from build123d import *

# Parameters (mm, degrees)
F1_DEPTH = 3.81
F3_DEPTH = 2.54
F5_DEPTH = 1.905


with BuildPart() as f1:
    # F0 (on Front) → F1 (new body)
    with BuildSketch(Plane.XZ):
        Polygon((-217.349024, 262.862362), (-255.449024, 262.862362), (-267.222571, 299.097615), (-278.996119, 262.862362), (-317.096119, 262.862362), (-286.272571, 240.467744), (-298.046119, 204.23249), (-267.222571, 226.627108), (-236.399024, 204.23249), (-248.172571, 240.467744), align=None)
    extrude(amount=F1_DEPTH)

    # F2 (on face) → F3 (join)
    with BuildSketch(Plane.XZ.offset(3.81)):
        Polygon((-239.378866, 208.333892), (-250.014215, 241.06613), (-222.17051, 261.295766), (-256.587222, 261.295766), (-267.222571, 294.028004), (-277.85792, 261.295766), (-312.274632, 261.295766), (-284.430927, 241.06613), (-295.066276, 208.333892), (-267.222571, 228.563528), align=None)
    extrude(amount=F3_DEPTH)

    # F4 (on face) → F5 (join)
    with BuildSketch(Plane.XZ.offset(6.35)):
        Polygon((-291.872742, 212.729414), (-267.222571, 230.638812), (-242.5724, 212.729414), (-251.987928, 241.707428), (-227.337756, 259.616826), (-257.807044, 259.616826), (-267.222571, 288.59484), (-276.638099, 259.616826), (-307.107386, 259.616826), (-282.457215, 241.707428), align=None)
    extrude(amount=F5_DEPTH)


solid = f1.part
For this review, take the finished solid that the model builds, in its own axes (mm). A direction names the side the tool comes from. Give positions to 0.01 mm unless a question says otherwise; leave off trailing zeros. Order: outer loops, then holes, each group sorted by start corner. A loop starts at its lowest first (then second) coordinate and runs counter-clockwise, first axis right, second up. Notation, with made-up numbers: M 25,48.25 L 55,48.25 A26 cw 55,85.25 Z; hole C 42.25,-10.5 d3. An arc over 180 degrees is marked long. Answer in a Markdown table with one row per item. Add a question column.
(1) Consider section B-B on y = -5. State the section outline as (x, z) points, and give its area (3 significant figures).
(2) Consider section A-A on x = -244.5. State the section outline as (y, z) points (3 decimals), and give its area (3 significant figures).
(3) Wall thickness on probe 1 along Y at (x, z) = (-269, 285.5); probe 2 along Y at (x, z) = (-231.5, 253.5); probe 3 along X at (y, z) = (-5.75, 217): over which ranges is each line inside the solid? List them lowest first. Write a range as [from, to].
(4) For faces 1 (the face through (-295, -5, 261.296)), 2 (the face through (-281.339, -5.062, 218.307)), 3 (the face through (-298, -2, 262.862)), list the 3-axis set-ups (+Z, -Z, +X, -X, +Y, -Y) from which the entire face can be reached by the end or side of a thin tool; tool diameter is ignored.
(5) Consider section C-C on z = 215. State the section outline as (x, y) points (3 decimals), and give its area (3 significant figures).
(6) Consider section D-D on x = -306. State the section outline as (y, z) points (3 decimals).
(7) For pin 1 (1.5 mm diameter, centred on x = -240, y = -7, fed in from +Z); pin 2 (0.6 mm diameter, centred on x = -295, y = -7, fed in from +Z); pin 3 (12 mm diameter, centred on x = -244, z = 265.5, fed in from -Y) (3 decimals); pin 4 (4 mm diameter, centred on x = -235.5, y = -2.5, fed in from +Z), all flat-tipped, find the tip position at first contact; note any pin that passes through.
(8) Mouldability with a two-part tool opening along X and no side actions: class faces 4 (the face through (-239, -5, 261.296)), 5 (the face through (-298.548, -5.062, 251.323)), 6 (the face through (-252.03, -1.88, 215.59)), 7 (the face through (-247.214, -7.289, 227.016)) as +X half, -X half, draft (parallel to the pull), parting line (faces both ways), or undercut.
Evaluation:
| question | item | result |
|---|---|---|
| 1 | outline | M -312.27,261.3 L -284.43,241.07 L -295.07,208.33 L -267.22,228.56 L -239.38,208.33 L -250.01,241.07 L -222.17,261.3 L -256.59,261.3 L -267.22,294.03 L -277.86,261.3 Z |
| 1 | area | 2,520 mm^2 |
| 2 | outline | M -8.255,214.13 L -6.35,214.13 L -6.35,212.055 L -3.81,212.055 L -3.81,210.118 L 0,210.118 L 0,229.165 L -3.81,229.165 L -3.81,224.095 L -6.35,224.095 L -6.35,218.662 L -8.255,218.662 Z; M -8.255,247.148 L -6.35,247.148 L -6.35,245.072 L -3.81,245.072 L -3.81,243.136 L 0,243.136 L 0,262.862 L -3.81,262.862 L -3.81,261.296 L -6.35,261.296 L -6.35,259.617 L -8.255,259.617 Z |
| 2 | area | 252 mm^2 |
| 3 | probe 1 | y = [-6.35, 0] |
| 3 | probe 2 | y = [-3.81, 0] |
| 3 | probe 3 | x = [-292.25, -283.14], [-251.31, -242.19] |
| 4 | face 1 | +Z, -X, -Y |
| 4 | face 2 | -Z, -Y |
| 4 | face 3 | +Z, -X, +Y, -Y |
| 5 | outline | M -294.548,-3.81 L -292.9,-3.81 L -292.9,-6.35 L -291.135,-6.35 L -291.135,-8.255 L -288.748,-8.255 L -288.748,-6.35 L -285.891,-6.35 L -285.891,-3.81 L -283.226,-3.81 L -283.226,0 L -294.548,0 Z; M -251.219,-3.81 L -248.554,-3.81 L -248.554,-6.35 L -245.698,-6.35 L -245.698,-8.255 L -243.31,-8.255 L -243.31,-6.35 L -241.545,-6.35 L -241.545,-3.81 L -239.898,-3.81 L -239.898,0 L -251.219,0 Z |
| 5 | area | 131 mm^2 |
| 6 | outline | M -8.255,258.812 L -6.35,258.812 L -6.35,256.737 L -3.81,256.737 L -3.81,254.801 L 0,254.801 L 0,262.862 L -3.81,262.862 L -3.81,261.296 L -6.35,261.296 L -6.35,259.617 L -8.255,259.617 Z |
| 7 | pin 1 | stops at z = 261.3 |
| 7 | pin 2 | stops at z = 259.62 |
| 7 | pin 3 | stops at y = -8.255 |
| 7 | pin 4 | stops at z = 262.86 |
| 8 | face 4 | draft |
| 8 | face 5 | -X half |
| 8 | face 6 | undercut |
| 8 | face 7 | +X half |
